Could you check a few things on this drawing? It's one solid part, dimensions in mm from its lowest x, y, z. A direction names the side the tool comes from. Coordinates: 2 decimals unless noted, no trailing zeros. Order: outer loops, then holes, each group sorted by start corner. A loop starts at its lowest first (then second) coordinate and runs counter-clockwise, first axis right, second up. Notation, with made-up numbers: (23, 62.25) - (64, 62.25) arc R14 cw to (64, 85.25) - close; hole circle Ø11 at (44.25, 8.5). An arc over 180 degrees is marked (long way). Return JSON: item names as keys, results as strings. Group by question number.
1) If we mould it in two halves opening along X, with no side actions, what happens to the marked faces 1, 2 and 3? For each: pulls with the +X half, pulls with the -X half, needs draft (parallel to the pull), parting line crosses it, or undercut.
2) Imagine slicing it at D-D (z = 12.75). Write out the boundary of the cut face in (x, y).
3) For pin 1 Ø3 at (x, z) = (3, 9.5) entering from -Y; pin 2 Ø1 at (y, z) = (3, 1) entering from -X; pin 3 Ø0.6 at (y, z) = (4, 1.5) entering from +X; pin 4 Ø1 at (x, z) = (6, 3.5) entering from -Y, each with a flat end and sliding along its axis, tell me the tip position at first contact or that it passes through.
4) Imagine slicing it at A-A (y = 3.5). Write out the boundary of the cut face in (x, z).
5) Imagine slicing it at C-C (z = 3). Write out the boundary of the cut face in (x, y).
6) If I drill on line 1 along Z through (x, y) = (3.75, 4.5); line 2 along Z through (x, y) = (3.25, 0.5); line 3 along Y through (x, z) = (5, 1), over which ranges is the centre line in solid material (lowest first)?
7) Imagine slicing it at B-B (x = 2.5). Write out the boundary of the cut face in (y, z).
8) Which directions (+Z, -Z, +X, -X, +Y, -Y) give clear straight access to the entire face, cutting with the end or side of a thin tool? Please do the marked faces 4, 5 and 6.
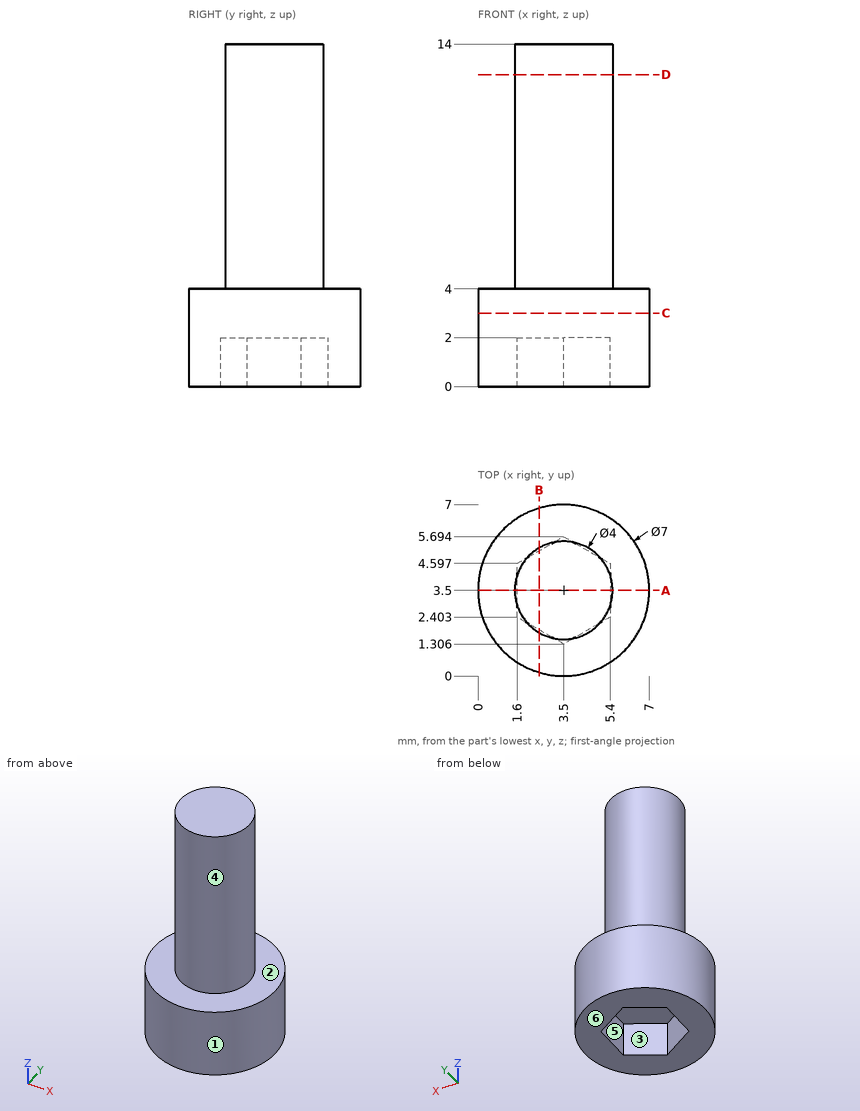
Calculated:
{
 "1": {"face 1": "parting line crosses it", "face 2": "needs draft", "face 3": "undercut"},
 "2": {"outline": "circle Ø4 at (3.5, 3.5)"},
 "3": {"pin 1": "y = 1.5", "pin 2": "x = 0", "pin 3": "x = 6.99", "pin 4": "y = 0.63"},
 "4": {"outline": "(0, 0) - (1.6, 0) - (1.6, 2) - (5.4, 2) - (5.4, 0) - (7, 0) - (7, 4) - (5.5, 4) - (5.5, 14) - (1.5, 14) - (1.5, 4) - (0, 4) - close"},
 "5": {"outline": "circle Ø7 at (3.5, 3.5)"},
 "6": {"line 1": "2 to 14", "line 2": "0 to 4", "line 3": "0.34 to 2.17, 4.83 to 6.66"},
 "7": {"outline": "(0.15, 0) - (1.88, 0) - (1.88, 2) - (5.12, 2) - (5.12, 0) - (6.85, 0) - (6.85, 4) - (5.23, 4) - (5.23, 14) - (1.77, 14) - (1.77, 4) - (0.15, 4) - close"},
 "8": {"face 4": "+Z", "face 5": "-Z", "face 6": "-Z, +X, -X, +Y, -Y"}
}
